Autodesk Inventor part; units mm, degrees
ref_plane "YZ Plane" through (0, 0, 0) normal (1, 0, 0) x (0, 1, 0)
ref_plane "XZ Plane" through (0, 0, 0) normal (0, 1, 0) x (-1, 0, 0)
ref_plane "XY Plane" through (0, 0, 0) normal (0, 0, 1) x (1, 0, 0)
sketch "스케치1" plane through (0, 0, 0) normal (0, 0, 1) x (1, 0, 0)
  line L0 (-9.7, -10) -> (9.7, -10)
  line L1 (10, -9.7) -> (10, 9.7)
  line L2 (9.7, 10) -> (-9.7, 10)
  line L3 (-10, 9.7) -> (-10, -9.7)
  line L4 (-10, -10) -> (10, 10) construction
  line L5 (10, -10) -> (-10, 10) construction
  circle A0 centre (-7, 7) radius 2
  line L6 (0, 15.6683) -> (0, -20)
  line L7 (-22.0072, 0) -> (22.0072, 0)
  circle A1 centre (0, 0) radius 2.15
  arc A2 (-9.7, 10) -> (-10, 9.7) centre (-9.7, 9.7) ccw
  arc A3 (10, 9.7) -> (9.7, 10) centre (9.7, 9.7) ccw
  arc A4 (9.7, -10) -> (10, -9.7) centre (9.7, -9.7) ccw
  arc A5 (-10, -9.7) -> (-9.7, -10) centre (-9.7, -9.7) ccw
  line L8 (-2.65, 10) -> (-2.65, 8.5)
  line L9 (-2.65, 8.5) -> (-4.15, 8.5)
  line L10 (-4.15, 8.5) -> (-4.15, 4.8)
  line L11 (4.15, 4.8) -> (4.15, 8.5)
  line L12 (4.15, 8.5) -> (2.65, 8.5)
  line L13 (2.65, 8.5) -> (2.65, 10)
  line L14 (-0.1, 3.3008) -> (0, 3.2)
  line L15 (0.1, 3.3008) -> (0, 3.2)
  arc A6 (-4.15, 4.8) -> (-0.1, 3.3008) centre (0, 9.7908) ccw
  arc A7 (0.1, 3.3008) -> (4.15, 4.8) centre (0, 9.7908) ccw
  circle A8 centre (7, 7) radius 2
  circle A9 centre (-7, -7) radius 2
  circle A10 centre (7, -7) radius 2
  line L16 (-3.3008, 0.1) -> (-3.2, 0)
  line L17 (-3.3008, -0.1) -> (-3.2, 0)
  arc A11 (-4.8, -4.15) -> (-3.3008, -0.1) centre (-9.7908, 0) ccw
  line L18 (-8.5, -4.15) -> (-4.8, -4.15)
  line L19 (-10, -2.65) -> (-8.5, -2.65)
  line L20 (-8.5, 2.65) -> (-10, 2.65)
  arc A12 (-3.3008, 0.1) -> (-4.8, 4.15) centre (-9.7908, 0) ccw
  line L21 (-4.8, 4.15) -> (-8.5, 4.15)
  line L22 (-8.5, 4.15) -> (-8.5, 2.65)
  line L23 (-8.5, -2.65) -> (-8.5, -4.15)
  line L24 (-0.1, -3.3008) -> (0, -3.2)
  line L25 (0.1, -3.3008) -> (0, -3.2)
  arc A13 (4.15, -4.8) -> (0.1, -3.3008) centre (0, -9.7908) ccw
  line L26 (4.15, -8.5) -> (4.15, -4.8)
  line L27 (2.65, -10) -> (2.65, -8.5)
  line L28 (-2.65, -8.5) -> (-2.65, -10)
  arc A14 (-0.1, -3.3008) -> (-4.15, -4.8) centre (0, -9.7908) ccw
  line L29 (-4.15, -4.8) -> (-4.15, -8.5)
  line L30 (-4.15, -8.5) -> (-2.65, -8.5)
  line L31 (2.65, -8.5) -> (4.15, -8.5)
  line L32 (3.3008, -0.1) -> (3.2, 0)
  line L33 (3.3008, 0.1) -> (3.2, 0)
  arc A15 (4.8, 4.15) -> (3.3008, 0.1) centre (9.7908, 0) ccw
  line L34 (8.5, 4.15) -> (4.8, 4.15)
  line L35 (10, 2.65) -> (8.5, 2.65)
  line L36 (8.5, -2.65) -> (10, -2.65)
  arc A16 (3.3008, -0.1) -> (4.8, -4.15) centre (9.7908, 0) ccw
  line L37 (4.8, -4.15) -> (8.5, -4.15)
  line L38 (8.5, -4.15) -> (8.5, -2.65)
  line L39 (8.5, 2.65) -> (8.5, 4.15)
  point P0 (2.65, 9.25)
  point P1 (-2.65, 9.25)
  point P2 (-4.15, 6.65)
  point P3 (0, 3.3)
  point P4 (-3.3, 0)
  point P5 (-9.25, -2.65)
  point P6 (-6.65, -4.15)
  point P7 (-9.25, 2.65)
  point P8 (0, -3.3)
  point P9 (2.65, -9.25)
  point P10 (4.15, -6.65)
  point P11 (-2.65, -9.25)
  point P12 (3.3, 0)
  point P13 (9.25, 2.65)
  point P14 (6.65, 4.15)
  point P15 (9.25, -2.65)
  dimension "d0" = 20
  dimension "d1" = 20
  dimension "d2" = 4
  dimension "d3" = 14
  dimension "d4" = 14
  dimension "d5" = 4.3
  dimension "d6" = 0.3
  dimension "d9" = 8.3
  dimension "d10" = 5.3
  dimension "d11" = 5.3
  dimension "d12" = 1.5
  dimension "d15" = 0.1
  dimension "d16" = 0.1
  dimension "d17" = 0.1
  dimension "d19" = 3.7
  dimension "d22" = 360
extrude "프로파일 길이 설정" add sketch "스케치1" along normal blind 500 contours A5 L3 L19 L23 L18 A11 L17 L7 A1 L6 L24 A14 L29 L30 L28 L0 | L27 L31 L26 A13 L25 L6 A1 L7 L32 A16 L37 L38 L36 L1 A4 L0 | L3 A2 L2 L8 L9 L10 A6 L14 L6 A1 L7 L16 A12 L21 L22 L20 | A1 L6 L15 A7 L11 L12 L13 L2 A3 L1 L35 L39 L34 A15 L33 L7
fillet "모서리" radius 0.05 32 edges at (10, 2.65, 250) (8.5, 2.65, 250) (8.5, 4.15, 250) (10, -2.65, 250) (8.5, -2.65, 250) (8.5, -4.15, 250) (2.65, 8.5, 250) (2.65, 10, 250) (4.15, 8.5, 250) (-4.15, 8.5, 250) (-2.65, 8.5, 250) (-2.65, 10, 250) (-10, 2.65, 250) (-8.5, 2.65, 250) (-8.5, 4.15, 250) (-8.5, -4.15, 250) (-8.5, -2.65, 250) (-10, -2.65, 250) (-2.65, -10, 250) (-2.65, -8.5, 250) (-4.15, -8.5, 250) (2.65, -8.5, 250) (4.15, -8.5, 250) (2.65, -10, 250) (4.15, -4.8, 250) (-4.15, -4.8, 250) (-4.8, -4.15, 250) (-4.8, 4.15, 250) (-4.15, 4.8, 250) (4.15, 4.8, 250) (4.8, -4.15, 250) (4.8, 4.15, 250)
equation "\"d0\" = d1"
equation "\"d11\" = d10"
properties part number "500mm 20x20 Profile"
Work out the finished part from the listing and answer in its coordinate system (mm). Give positions to 0.01 mm unless a question says otherwise; leave off trailing zeros. Write item = value, one per line. Start each with the question number.
(1) Find the intervals of material crossed by probe 1 along Y at (x, z) = (-7, 312.5); probe 2 along X at (y, z) = (-7.25, 234.5); probe 3 along X at (y, z) = (5.25, 435.5), in increasing order. Write a range as from..to.
(2) Given pin 1 Ø2.5 at (x, y) = (7, -7) entering from -Z; pin 2 Ø4 at (y, z) = (0, 364.5) entering from -X, each flat-ended and moving along its own axis, determine where each tip first touches the part or whether it passes through.
(3) Find section A-A on z = 171. Give the number of separate pieces and of enclosed holes in the cut face, and give its area (3 significant figures).
From the geometry:
q1.probe_1 = -10..-9, -5..-4.15, 4.15..5, 9..10
q1.probe_2 = -10..-8.98, -5.02..-4.15, 4.15..5.02, 8.98..10
q1.probe_3 = -10..-7.97, -6.03..-4.15, 4.15..6.03, 7.97..10
q2.pin_1 = through
q2.pin_2 = -3.62
q3.separate_pieces = 1
q3.enclosed_holes = 5
q3.area = 146 mm^2
